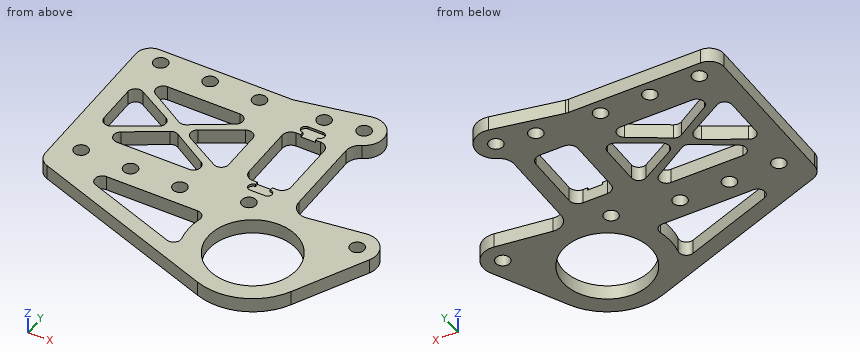
```python
from build123d import *

# Parameters (mm, degrees)
SKETCH_2_R          = 9
SKETCH_2_R_2        = 1.45
EXTRUDE_1_DEPTH     = 3
EXTRUDE_START       = -3
SKETCH_4_R          = 1.45
EXTRUDE_2_DEPTH     = 3
SKETCH_5_R          = 1.45
SKETCH_5_W          = 8.5
SKETCH_5_H          = 15
EXTRUDE_3_DEPTH     = 3
SKETCH_6_W          = 3
SKETCH_6_H          = 20
CUT_EXTRUDE_2_DEPTH = 0.5
SKETCH_7_R          = 1.45
CUT_EXTRUDE_3_DEPTH = 20
FILLET_1_R          = 1.8
FILLET_2_R          = 3
SKETCH_8_R          = 0.9
CUT_EXTRUDE_4_DEPTH = 0.5
CUT_EXTRUDE_5_DEPTH = 10.5
FILLET_3_R          = 1.5


with BuildPart() as part:
    # 草图2 → 凸台-拉伸1 (new body)
    with BuildSketch(Plane.XY):
        with BuildLine():
            Line((-10, -7), (-10, -16.423561614))
            Line((-10, -16.423561614), (30.724748208, -31.24615776))
            ThreePointArc((30.724748208, -31.24615776), (47.310096913, -21.670602221), (35, -7))
            Line((35, -7), (-10, -7))
        make_face()
        with Locations((35, -19.5)):
            Circle(SKETCH_2_R, mode=Mode.SUBTRACT)
        with Locations((15, -10.5)):
            Circle(SKETCH_2_R_2, mode=Mode.SUBTRACT)
        with Locations((5, -10.5)):
            Circle(SKETCH_2_R_2, mode=Mode.SUBTRACT)
        with Locations((-5, -10.5)):
            Circle(SKETCH_2_R_2, mode=Mode.SUBTRACT)
    extrude(amount=EXTRUDE_1_DEPTH)

    # 草图4 → 凸台-拉伸2 (add)
    with BuildSketch(Plane.XY.offset(3).offset(EXTRUDE_START)):
        with BuildLine():
            Line((35, -7), (49.461817276, -5.036370432))
            ThreePointArc((49.461817276, -5.036370432), (53.268884157, -6.694702543), (53.552947171, -10.837543578))
            Line((53.552947171, -10.837543578), (46.102959909, -25.24232368))
            ThreePointArc((46.102959909, -25.24232368), (45.677758332, -13.00111725), (35, -7))
        make_face()
        with Locations((50, -9)):
            Circle(SKETCH_4_R, mode=Mode.SUBTRACT)
    extrude(amount=EXTRUDE_2_DEPTH)

    # 草图5 → 凸台-拉伸3 (add)
    with BuildSketch(Plane(origin=(0, 0, 0), x_dir=(-1, 0, 0), z_dir=(0, 0, -1))):
        with BuildLine():
            Line((-35, -7), (-35, 15))
            ThreePointArc((-35, 15), (-38.979463437, 19.404809528), (-34.194537642, 22.918064623))
            Line((-34.194537642, 22.918064623), (-20, 20))
            Line((-20, 20), (10, 20))
            Line((10, 20), (10, -7))
            Line((10, -7), (-35, -7))
        make_face()
        with Locations((-35, 19)):
            Circle(SKETCH_5_R, mode=Mode.SUBTRACT)
        with Locations((-27.5, 5)):
            Rectangle(SKETCH_5_W, SKETCH_5_H, mode=Mode.SUBTRACT)
    extrude(amount=-EXTRUDE_3_DEPTH)

    # 草图6 → 切除-拉伸2 (cut)
    with BuildSketch(Plane.XY.offset(3)):
        with Locations((27.5, 5)):
            Rectangle(SKETCH_6_W, SKETCH_6_H)
    extrude(amount=-CUT_EXTRUDE_2_DEPTH, mode=Mode.SUBTRACT)

    # 草图7 → 切除-拉伸3 (cut)
    with BuildSketch(Plane.XY.offset(3)):
        with Locations((27.5, 18)):
            Circle(SKETCH_7_R)
        with Locations(Location((27.5, -8, 0), (0, 0, 180))):
            Circle(SKETCH_7_R)
        with Locations((-5, 17)):
            Circle(SKETCH_7_R)
        with Locations((5, 17)):
            Circle(SKETCH_7_R)
        with Locations((15, 17)):
            Circle(SKETCH_7_R)
    extrude(amount=-CUT_EXTRUDE_3_DEPTH, mode=Mode.SUBTRACT)

    # 圆角1
    fillet_1_edges = [part.edges().sort_by_distance(p)[0] for p in [
        (31.75, 12.5, 1.5),
        (23.25, 12.5, 1.5),
        (23.25, -2.5, 1.5),
        (31.75, -2.5, 1.5),
    ]]
    fillet(fillet_1_edges, radius=FILLET_1_R)

    # 圆角2
    fillet_2_edges = [part.edges().sort_by_distance(p)[0] for p in [
        (35, 15, 1.5),
        (20, 20, 1.5),
        (-10, 20, 1.5),
        (35, -7, 1.5),
        (-10, -16.423561614, 1.5),
    ]]
    fillet(fillet_2_edges, radius=FILLET_2_R)

    # 草图8 → 切除-拉伸4 (cut)
    with BuildSketch(Plane.XY.offset(3)):
        with Locations((26, 14.1)):
            Circle(SKETCH_8_R)
        with Locations((29, 14.1)):
            Circle(SKETCH_8_R)
        with Locations((26, -4.1)):
            Circle(SKETCH_8_R)
        with Locations((29, -4.1)):
            Circle(SKETCH_8_R)
    extrude(amount=-CUT_EXTRUDE_4_DEPTH, mode=Mode.SUBTRACT)

    # 草图9 → 切除-拉伸5 (cut)
    with BuildSketch(Plane(origin=(0, 0, 0), x_dir=(-1, 0, 0), z_dir=(0, 0, -1))):
        Polygon((-6.625, 4.25), (-19.25, 12), (6, 12), align=None)
        Polygon((-7.625, 3.25), (-19.25, 10), (-19.25, -3.5), align=None)
        Polygon((6, 10), (6, -3.5), (-5.625, 3.25), align=None)
        Polygon((-19.25, -5.5), (6, -5.5), (-6.625, 2.25), align=None)
        with BuildLine():
            Line((-23, -14.5), (6, -14.5))
            Line((6, -14.5), (-23.298682976, -25.163848506))
            ThreePointArc((-23.298682976, -25.163848506), (-22.005096252, -19.863973337), (-23, -14.5))
        make_face()
    extrude(amount=-CUT_EXTRUDE_5_DEPTH, mode=Mode.SUBTRACT)

    # 圆角3
    fillet_3_edges = [part.edges().sort_by_distance(p)[0] for p in [
        (7.625, 3.25, 1.5),
        (19.25, -3.5, 1.5),
        (19.25, 10, 1.5),
        (23.298682976, -25.163848506, 1.5),
        (23, -14.5, 1.5),
        (-6, -14.5, 1.5),
        (19.25, -5.5, 1.5),
        (6.625, 2.25, 1.5),
        (-6, -5.5, 1.5),
        (5.625, 3.25, 1.5),
        (-6, 10, 1.5),
        (-6, -3.5, 1.5),
        (-6, 12, 1.5),
        (6.625, 4.25, 1.5),
        (19.25, 12, 1.5),
    ]]
    fillet(fillet_3_edges, radius=FILLET_3_R)


solid = part.part
```
Design review of the part built by this model. Coordinates are the model's own, in mm. Give positions to 0.01 mm unless a question says otherwise; leave off trailing zeros. Order: outer loops, then holes, each group sorted by start corner. A loop starts at its lowest first (then second) coordinate and runs counter-clockwise, first axis right, second up. Notation, with made-up numbers: (4.5, 84) -> (45.5, 84) arc R9 ccw to (45.5, 98) -> close; hole circle Ø2 at (43.25, 80.25). An arc over 180 degrees is marked (long way). Write item = value, one per line. Start each with the question number.
(1) We need section A-A on y = -19.5. Write out the cut boundary in (x, z).
(2) For pin 1 (4.5 mm diameter, centred on x = 35, y = 19, fed in from +Z); pin 2 (1 mm diameter, centred on y = -4, z = 2, fed in from +X); pin 3 (1.7 mm diameter, centred on x = 5, y = 17, fed in from +Z); pin 4 (0.9 mm diameter, centred on x = 11.5, z = 1.5, fed in from +Y), all flat-tipped, find the tip position at first contact; note any pin that passes through.
(3) We need section C-C on x = 45. Write out the cut boundary in (y, z), plus the area to 3 significant figures.
(4) We need section B-B on z = 1.4. State how many separate pieces and enclosed holes the cut face has, plus the area to 3 significant figures.
(5) To check wall thickness, follow line 1 along Y through (x, z) = (3.5, 0.25); line 2 along X through (y, z) = (-17, 1.1); line 3 along Y through (x, z) = (-5, 1.5). State the ranges of each line that lie inside material, in increasing order.
Numbers:
q1.outline = (-1.55, 0) -> (7.74, 0) -> (7.74, 3) -> (-1.55, 3) -> close; (22, 0) -> (26, 0) -> (26, 3) -> (22, 3) -> close; (44, 0) -> (49.07, 0) -> (49.07, 3) -> (44, 3) -> close
q2.pin_1 = 3
q2.pin_2 = 35.15
q2.pin_3 = through
q2.pin_4 = 20
q3.outline = (-27, 0) -> (-5.64, 0) -> (-5.64, 3) -> (-27, 3) -> close
q3.area = 64.1 mm^2
q4.separate_pieces = 1
q4.enclosed_holes = 17
q4.area = 1,510 mm^2
q5.line_1 = -21.34 to -17.96, -14.5 to -5.5, 0.33 to 2.02, 4.48 to 6.17, 12 to 20
q5.line_2 = -8.35 to 1.39, 22.24 to 26.35, 43.65 to 50.37
q5.line_3 = -18.24 to -11.95, -9.05 to -2.31, 8.81 to 15.55, 18.45 to 20
